CAD build for the part. Positions are in the model's coordinates, mm. A direction names the side the tool comes from. Round coordinates to 2 decimals unless told otherwise and drop trailing zeros. Write each loop counter-clockwise with the first axis right and the second up, starting at its lowest first coordinate (ties: lowest second). Pieces come first, ordered by that corner, then holes. Notation, with made-up numbers: (-1, 18.25) -> (20, 18.25) arc R13 ccw to (20, 36.25) -> close; hole circle Ø8 at (68.5, 39.5). An arc over 180 degrees is marked (long way). Put each result on its own line as item: value. Start each with the question number.
1. Saw through at D-D on x = -17. List the corners of the cut face in (y, z), and give its area (3 significant figures).
2. 3-axis set-ups, long thin cutter, end or side, ignore diameter. For faces 4 (the flat face through (-22, 7.8, 2)), 5 (the cylindrical face through (-27.14, 0.9, 2.03)), 6 (the flat face through (-20, 11.8, 2)): which of +Z, -Z, +X, -X, +Y, -Y reach the whole face in a straight line?
3. Saw through at A-A on x = -22.25. List the corners of the cut face in (y, z).
4. Pull direction Y, two halves, no side cores. Call faces 1 (the flat face through (-11, 13, 0)), 2 (the cylindrical face through (-14.1, 32.94, 2.03)), 3 (the flat face through (-18, 6, 2)): pulls with the +Y half, pulls with the -Y half, needs draft (parallel to the pull), parting line crosses it, or undercut.
5. Saw through at C-C on y = 19. List the corners of the cut face in (x, z), and give its area (3 significant figures).
6. Flat gauge pins, fed straight in: P1, Ø1.1, axis at y = 6.5, z = 3, coming from the -X side; P2, Ø2, axis at y = 11, z = 3.5, coming from the -X side; P3, Ø1.5, axis at x = -15.5, z = 3, coming from the +Y side. Where does each tip first touch, or does it go through?
7. Drill centre lines: line 1 (Y direction, x = -23.5, z = 3.5); line 2 (X direction, y = 15.5, z = 1.5); line 3 (Y direction, x = -6.5, z = 1.9). Where is each one in solid material? Low to high. Write a range as from..to.
from build123d import *

# Parameters (mm, degrees)
ESTRUSIONE_ESTRUSIONE1_DEPTH = 4
RACCORDO1_R                  = 1
RACCORDO2_R                  = 3
RACCORDO3_R                  = 5
RACCORDO4_R                  = 15


with BuildPart() as part:
    # Schizzo1 → Estrusione-Estrusione1 (new body)
    with BuildSketch(Plane.XY):
        Polygon((-15, 33.8), (0, 33.8), (0, 0), (-28, 0), (-28, 4), (-18, 4), (-18, 7.8), (-28, 7.8), (-28, 11.8), (-15, 11.8), (-15, 26), (-5, 26), (-5, 29.8), (-15, 29.8), align=None)
    extrude(amount=ESTRUSIONE_ESTRUSIONE1_DEPTH)

    # Raccordo1
    raccordo1_edges = [part.edges().sort_by_distance(p)[0] for p in [
        (-28, 4, 2),
        (-28, 7.8, 2),
        (-15, 26, 2),
        (-15, 29.8, 2),
    ]]
    fillet(raccordo1_edges, radius=RACCORDO1_R)

    # Raccordo2
    raccordo2_edges = [part.edges().sort_by_distance(p)[0] for p in [
        (-28, 0, 2),
        (-28, 11.8, 2),
        (-15, 33.8, 2),
    ]]
    fillet(raccordo2_edges, radius=RACCORDO2_R - 0.0001)  # a hair under: the kernel refuses the full size

    # Raccordo3
    raccordo3_edges = [part.edges().sort_by_distance(p)[0] for p in [
        (0, 33.8, 2),
    ]]
    fillet(raccordo3_edges, radius=RACCORDO3_R)

    # Raccordo4
    raccordo4_edges = [part.edges().sort_by_distance(p)[0] for p in [
        (0, 0, 2),
    ]]
    fillet(raccordo4_edges, radius=RACCORDO4_R)


solid = part.part
Return value:
1. outline: (0, 0) -> (11.8, 0) -> (11.8, 4) -> (0, 4) -> close
1. area: 47.2 mm^2
2. face 4: +Z, -Z, -X
2. face 5: +Z, -Z, -X, -Y
2. face 6: +Z, -Z, -X, +Y
3. outline: (0, 0) -> (4, 0) -> (4, 4) -> (0, 4) -> close; (7.8, 0) -> (11.8, 0) -> (11.8, 4) -> (7.8, 4) -> close
4. face 1: needs draft
4. face 2: pulls with the +Y half
4. face 3: undercut
5. outline: (-15, 0) -> (0, 0) -> (0, 4) -> (-15, 4) -> close
5. area: 60.0 mm^2
6. P1: stops at x = -18
6. P2: stops at x = -27.75
6. P3: stops at y = 32
7. line 1: y = 0..4, 7.8..11.8
7. line 2: x = -15..0
7. line 3: y = 2.64..26, 29.8..33.8
